from build123d import *

# Parameters (mm, degrees)
BOSS_EXTRUDE2_DEPTH = 30


with BuildPart() as part:
    # Sketch1 → Boss-Extrude2 (new body)
    with BuildSketch(Plane.XY):
        with BuildLine():
            Line((3, -8.5), (4.952380952, -5.5))
            Line((4.952380952, -5.5), (4.952380952, -4.5))
            Line((4.952380952, -4.5), (3, -4.5))
            Line((3, -4.5), (3, -2.5))
            Line((3, -2.5), (6.271768379, -2.5))
            Line((6.271768379, -2.5), (6.271768379, -6.5))
            Line((6.271768379, -6.5), (3.35255813, -10.985615749))
            ThreePointArc((3.35255813, -10.985615749), (0, -12.803792203), (-3.35255813, -10.985615749))
            Line((-3.35255813, -10.985615749), (-6.271768379, -6.5))
            Line((-6.271768379, -6.5), (-6.271768379, -2.5))
            Line((-6.271768379, -2.5), (-3, -2.5))
            Line((-3, -2.5), (-3, -4.5))
            Line((-3, -4.5), (-4.952380952, -4.5))
            Line((-4.952380952, -4.5), (-4.952380952, -5.5))
            Line((-4.952380952, -5.5), (-3, -8.5))
            Line((-3, -8.5), (-2.514418598, -9.246137277))
            ThreePointArc((-2.514418598, -9.246137277), (0, -10.609769618), (2.514418598, -9.246137277))
            Line((2.514418598, -9.246137277), (3, -8.5))
        make_face()
    extrude(amount=BOSS_EXTRUDE2_DEPTH)


solid = part.part
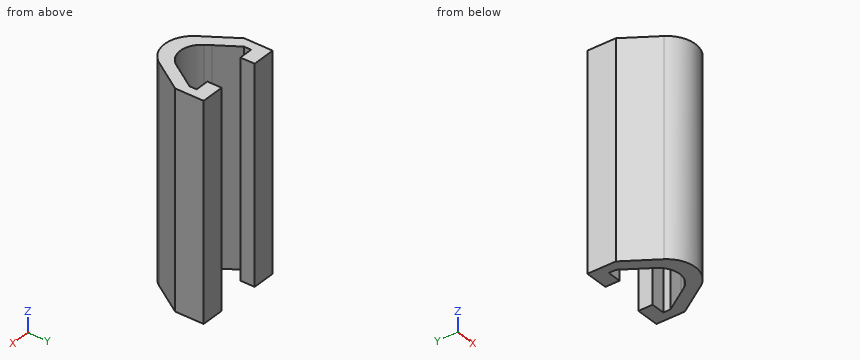
Geometry: final body of the model. Coordinates: model frame, mm. Give positions to 0.01 mm unless a question says otherwise; leave off trailing zeros. Loops run counter-clockwise (first coordinate to the right, second up) from the corner with the lowest first, then second, coordinate; pieces in that order, holes last. Notation, with made-up numbers: M -8,26 L 20,26 A16 cw 20,51 Z; hole C 22,77.5 d1. An arc over 180 degrees is marked long. Put each result on its own line as item: value.
1) Cut plane A-A, the plane y = -3.25. Return the cut outline in (x, z), plus the area to 3 significant figures.
Computed values:
outline: M -6.27,0 L -3,0 L -3,30 L -6.27,30 Z; M 3,0 L 6.27,0 L 6.27,30 L 3,30 Z
area: 196 mm^2
2) First-contact query: P1, Ø3, axis at x = 1.5, z = 7.5, coming from the -Y side; P2, Ø0.6, axis at x = 4, z = 20, coming from the -Y side; P3, Ø3, axis at x = 4, z = 26, coming from the -Y side; P4, Ø2, axis at x = -4, z = 7.5, coming from the -Y side. Flat tips, straight axial feed; report the tip coordinate or a pass-through.
Computed values:
P1: stops at y = -12.8
P2: stops at y = -10.45
P3: stops at y = -11.93
P4: stops at y = -11.45
3) Cut plane C-C, the plane x = -3.75. Return the cut outline in (y, z).
Computed values:
outline: M -10.37,0 L -7.35,0 L -7.35,30 L -10.37,30 Z; M -4.5,0 L -2.5,0 L -2.5,30 L -4.5,30 Z
4) Material intervals for L1, parallel to X at y = -5, z = 2.25; L2, parallel to X at y = -9.5, z = 23; L3, parallel to Y at x = -5.5, z = 18.5, sorted ascending. Write a range as from..to.
Computed values:
L1: x = -6.27..-4.95, 4.95..6.27
L2: x = -4.32..-2.33, 2.33..4.32
L3: y = -7.69..-2.5
5) Cut plane D-D, the plane y = -11.75. Return the cut outline in (x, z), plus the area to 3 significant figures.
Computed values:
outline: M -2.71,0 L 2.71,0 L 2.71,30 L -2.71,30 Z
area: 162 mm^2
6) Cut plane B-B, the plane z = 20.5. Return the cut outline in (x, y).
Computed values:
outline: M -6.27,-6.5 L -3.35,-10.99 A4 ccw 3.35,-10.99 L 6.27,-6.5 L 6.27,-2.5 L 3,-2.5 L 3,-4.5 L 4.95,-4.5 L 4.95,-5.5 L 2.51,-9.25 A3 cw -2.51,-9.25 L -4.95,-5.5 L -4.95,-4.5 L -3,-4.5 L -3,-2.5 L -6.27,-2.5 Z
